Geometry check sheet. Reference: the model listing, model coordinates, mm. Round coordinates to 2 decimals unless told otherwise and drop trailing zeros. Order: outer loops, then holes, each group sorted by start corner. A loop starts at its lowest first (then second) coordinate and runs counter-clockwise, first axis right, second up.
(1) Material ranges on line 1 along Y through (x, z) = (15, 7.25); line 2 along X through (y, z) = (13, 4.25); line 3 along X through (y, z) = (21.5, 4.5), recorded low to high.
(2) Sectioned sample at A-A (z = 1.5). Record the boundary of the cut face in (x, y), plus the area to 3 significant figures.
(3) Sectioned sample at D-D (z = 8). Record the boundary of the cut face in (x, y), plus the area to 3 significant figures.
(4) Go/stop test with flat-tipped pins: pin 1 (5 mm diameter, centred on y = 20.5, z = 3.5, fed in from -X); pin 2 (1.5 mm diameter, centred on y = 23.5, z = 5, fed in from +X); pin 3 (4 mm diameter, centred on y = 1.5, z = 9, fed in from +X). Record where each tip stops, or that it passes through.
from build123d import *

# Parameters (mm, degrees)
F1_DEPTH = 10
F2_SIZE  = 9.99999


# Not quite as in the source:
# - a fillet or chamfer is up to 0.001 mm smaller than in the source, because OpenCascade refuses the exact size


with BuildPart() as f1:
    # F0 (on Top) → F1 (new body)
    with BuildSketch(Plane.XY):
        with BuildLine():
            Line((-40, -60), (40, -60))
            ThreePointArc((40, -60), (54.1421356237, -54.1421356237), (60, -40))
            Line((60, -40), (60, 40))
            ThreePointArc((60, 40), (54.1421356237, 54.1421356237), (40, 60))
            Line((40, 60), (-40, 60))
            ThreePointArc((-40, 60), (-54.1421356237, 54.1421356237), (-60, 40))
            Line((-60, 40), (-60, -40))
            ThreePointArc((-60, -40), (-54.1421356237, -54.1421356237), (-40, -60))
        make_face()
    extrude(amount=F1_DEPTH)

    # F2 (size 10 in the source; OpenCascade refuses exactly that, so slightly less here)
    f2_edges = [f1.edges().sort_by_distance(p)[0] for p in [
        (-60, 0, 0),
    ]]
    chamfer(f2_edges, length=F2_SIZE)


solid = f1.part
Answer below:
1. line 1: y = -57.25 to 57.25
1. line 2: x = -54.25 to 54.25
1. line 3: x = -54.5 to 54.5
2. outline: (-51.5, -40) arc R11.5 ccw to (-40, -51.5) - (40, -51.5) arc R11.5 ccw to (51.5, -40) - (51.5, 40) arc R11.5 ccw to (40, 51.5) - (-40, 51.5) arc R11.5 ccw to (-51.5, 40) - close
2. area: 10,500 mm2
3. outline: (-58, -40) arc R18 ccw to (-40, -58) - (40, -58) arc R18 ccw to (58, -40) - (58, 40) arc R18 ccw to (40, 58) - (-40, 58) arc R18 ccw to (-58, 40) - close
3. area: 13,200 mm2
4. pin 1: stops at x = -56
4. pin 2: stops at x = 55.75
4. pin 3: stops at x = 60
